Work out the finished part from the listing and answer in its coordinate system (mm). A direction names the side the tool comes from. Round coordinates to 2 decimals unless told otherwise and drop trailing zeros. Write each loop counter-clockwise with the first axis right and the second up, starting at its lowest first coordinate (ties: lowest second). Pieces come first, ordered by that corner, then holes. Notation, with made-up numbers: (8.5, 87.5) -> (48.5, 87.5) arc R20 ccw to (48.5, 111.5) -> close; hole circle Ø10 at (22.25, 38). An arc over 180 degrees is marked (long way). Answer as a JSON object with one key per item and string values. Group by question number.
from build123d import *

# Parameters (mm, degrees)
PAD_DEPTH        = 20
HOLE_D           = 4
HOLE_DEPTH       = 25
HOLE_CSINK_D     = 8
HOLE_CSINK_ANGLE = 90


with BuildPart() as part:
    # Sketch → Pad (new body, symmetric)
    with BuildSketch(Plane.XY):
        Polygon((-13, -30.5), (13, -30.5), (13, 28), (10.5, 30.5), (10.5, 32.5), (12.5, 32.5), (15, 30), (15, -32.5), (-15, -32.5), (-15, 30), (-12.5, 32.5), (-10.5, 32.5), (-10.5, 30.5), (-13, 28), align=None)
    extrude(amount=PAD_DEPTH, both=True)

    # Hole
    with Locations(Plane(origin=(0, -30.5, 0), x_dir=(-1, 0, 0), z_dir=(0, 1, 0))):
        with Locations((0, 12), (0, -12)):
            CounterSinkHole(HOLE_D / 2, HOLE_CSINK_D / 2, depth=HOLE_DEPTH, counter_sink_angle=HOLE_CSINK_ANGLE)


solid = part.part
1) Straight lines are drawn through the part: L1, parallel to X at y = 1, z = 9.5; L2, parallel to Y at x = -9.5, z = 1; L3, parallel to Y at x = -2.25, z = 13. For each, find the intervals that lie inside material, in ascending order.
2) Each of these flat-tipped pins is pushed along its axis until it touches: P1, Ø8, axis at x = 4, z = 2.5, coming from the +Y side; P2, Ø0.6, axis at y = 31.5, z = -8.5, coming from the -X side; P3, Ø0.6, axis at y = 31, z = 3.5, coming from the +X side. Where does it stop, or does it pass through?
3) A cutting plane is placed at D-D on z = 0. Determine the outline of the cut face in (x, y).
4) A cutting plane is placed at A-A on x = 0. Determine the outline of the cut face in (y, z).
5) A cutting plane is placed at C-C on y = -23. Determine the outline of the cut face in (x, z).
6) A cutting plane is placed at B-B on z = 12. Determine the outline of the cut face in (x, y).
7) A tool of negligible diameter and unlimited length cuts with its end or side. For faces 1 (the face through (-12, 32.5, 0)), 2 (the face through (0, -30.5, 0)), 3 (the face through (10.5, 31, 0)), from which of +Z, -Z, +X, -X, +Y, -Y can it reach the whole face along a straight path? Write none if from no direction.
Established:
{
 "1": {"L1": "x = -15 to -13, 13 to 15", "L2": "y = -32.5 to -30.5", "L3": "y = -32.5 to -32.04"},
 "2": {"P1": "stops at y = -30.5", "P2": "stops at x = -13.8", "P3": "stops at x = 14.3"},
 "3": {"outline": "(-15, -32.5) -> (15, -32.5) -> (15, 30) -> (12.5, 32.5) -> (10.5, 32.5) -> (10.5, 30.5) -> (13, 28) -> (13, -30.5) -> (-13, -30.5) -> (-13, 28) -> (-10.5, 30.5) -> (-10.5, 32.5) -> (-12.5, 32.5) -> (-15, 30) -> close"},
 "4": {"outline": "(-32.5, -20) -> (-30.5, -20) -> (-30.5, -16) -> (-32.5, -14) -> close; (-32.5, -10) -> (-30.5, -8) -> (-30.5, 8) -> (-32.5, 10) -> close; (-32.5, 14) -> (-30.5, 16) -> (-30.5, 20) -> (-32.5, 20) -> close"},
 "5": {"outline": "(-15, -20) -> (-13, -20) -> (-13, 20) -> (-15, 20) -> close; (13, -20) -> (15, -20) -> (15, 20) -> (13, 20) -> close"},
 "6": {"outline": "(-15, -32.5) -> (-2, -32.5) -> (-4, -30.5) -> (-13, -30.5) -> (-13, 28) -> (-10.5, 30.5) -> (-10.5, 32.5) -> (-12.5, 32.5) -> (-15, 30) -> close; (2, -32.5) -> (15, -32.5) -> (15, 30) -> (12.5, 32.5) -> (10.5, 32.5) -> (10.5, 30.5) -> (13, 28) -> (13, -30.5) -> (4, -30.5) -> close"},
 "7": {"face 1": "+Z, -Z, +X, -X, +Y", "face 2": "+Z, -Z", "face 3": "+Z, -Z, +Y"}
}
